Can you work these out from the model? Positions are in its coordinate system, mm. A direction names the side the tool comes from. Coordinates: 2 decimals unless noted, no trailing zeros. Order: outer loops, then holes, each group sorted by start corner. A loop starts at its lowest first (then second) coordinate and runs counter-clockwise, first axis right, second up. Notation, with made-up numbers: (24, 22) -> (52, 22) arc R9 cw to (52, 26) -> close; hole circle Ø3 at (-6, 85.5). An arc over 180 degrees is marked (long way). Answer as a JSON object with one key per item and string values. Group by question number.
(1) I need wall thicknesses on line 1 (X direction, y = 0.45, z = 34); line 2 (X direction, y = 1.6, z = -27); line 3 (Z direction, x = 20, y = 0.95). Which ranges of each line are inside material? Lowest first, please.
(2) I want a section at A-A, the plane z = -4. List the corners of the cut face in (x, y) for me.
(3) For pin 1 (0.8 mm diameter, centred on x = -1.5, y = 0.5, fed in from +Z); pin 2 (0.8 mm diameter, centred on x = 6, y = 2, fed in from -Z); pin 3 (0.8 mm diameter, centred on x = -21.5, z = 18, fed in from +Y), each with a flat end and sliding along its axis, tell me the tip position at first contact or that it passes through.
(4) I want a section at D-D, the plane x = -4.5. List the corners of the cut face in (y, z) for me.
(5) Which directions (+Z, -Z, +X, -X, +Y, -Y) give clear straight access to the entire face, cutting with the end or side of a thin tool? Please do faces 1 (the flat face through (-22, 1, -9)), 2 (the cylindrical face through (0.62, -1.4, -51.93)), 3 (the flat face through (24, 1, 0)).
(6) I want a section at B-B, the plane y = 0.8. List the corners of the cut face in (x, z) for me.
(7) I want a section at C-C, the plane z = -27.5. List the corners of the cut face in (x, y) for me.
(8) If we mould it in two halves opening along Z, with no side actions, what happens to faces 4 (the flat face through (22, 1, -11)), 5 (the flat face through (12, 1, -47)), 6 (the flat face through (-24, 1, -2))? For each: pulls with the +Z half, pulls with the -Z half, needs draft (parallel to the pull), parting line crosses it, or undercut.
from build123d import *

# Parameters (mm, degrees)
BOSS_EXTRUDE1_DEPTH = 2.5
SKETCH4_W           = 40
SKETCH4_H           = 1.5
BOSS_EXTRUDE3_DEPTH = 1.5
SKETCH6_R           = 2
BOSS_EXTRUDE4_DEPTH = 10


with BuildPart() as part:
    # Sketch2 → Boss-Extrude1 (new body)
    with BuildSketch(Plane(origin=(0, 0, 0), x_dir=(1, 0, 0), z_dir=(0, 1, 0))):
        Polygon((-22, -45), (-22, 45), (22, 45), (22, -45), (24, -45), (24, 47), (-24, 47), (-24, -45), align=None)
    extrude(amount=BOSS_EXTRUDE1_DEPTH)

    # Sketch4 → Boss-Extrude3 (add)
    with BuildSketch(Plane(origin=(-22, 0, 0), x_dir=(0, 0, -1), z_dir=(1, 0, 0))):
        Polygon((45, 1.75), (15, 1.75), (45, 2.5), align=None)
        with Locations((-25, 0.75)):
            Rectangle(SKETCH4_W, SKETCH4_H)
    boss_extrude3 = extrude(amount=BOSS_EXTRUDE3_DEPTH)

    # Mirror1: Boss-Extrude3 across plane
    add(boss_extrude3.mirror(Plane(origin=(0, 0, 0), x_dir=(0, 0, 1), z_dir=(1, 0, 0))))

    # Sketch6 → Boss-Extrude4 (add)
    with BuildSketch(Plane(origin=(0, 0, -47), x_dir=(-1, 0, 0), z_dir=(0, 0, -1))):
        with Locations(Location((0, 0.5, 0), (0, 0, 194.477512186))):
            Circle(SKETCH6_R)
    extrude(amount=BOSS_EXTRUDE4_DEPTH)


solid = part.part
Computed values:
{
 "1": {"line 1": "x = -24 to -20.5, 20.5 to 24", "line 2": "x = -24 to -22, 22 to 24", "line 3": "z = -47 to -45"},
 "2": {"outline": "(-24, 0) -> (-22, 0) -> (-22, 2.5) -> (-24, 2.5) -> close; (22, 0) -> (24, 0) -> (24, 2.5) -> (22, 2.5) -> close"},
 "3": {"pin 1": "stops at z = -45", "pin 2": "stops at z = -47", "pin 3": "stops at y = 1.5"},
 "4": {"outline": "(0, -47) -> (2.5, -47) -> (2.5, -45) -> (0, -45) -> close"},
 "5": {"face 1": "none", "face 2": "-Z", "face 3": "+Z, -Z, +X, +Y, -Y"},
 "6": {"outline": "(-24, -47) -> (-1.98, -47) -> (-1.98, -57) -> (1.98, -57) -> (1.98, -47) -> (24, -47) -> (24, 45) -> (20.5, 45) -> (20.5, 5) -> (22, 5) -> (22, -45) -> (-22, -45) -> (-22, 5) -> (-20.5, 5) -> (-20.5, 45) -> (-24, 45) -> close"},
 "7": {"outline": "(-24, 0) -> (-22, 0) -> (-22, 1.75) -> (-20.5, 1.75) -> (-20.5, 2.06) -> (-22, 2.06) -> (-22, 2.5) -> (-24, 2.5) -> close; (20.5, 1.75) -> (22, 1.75) -> (22, 0) -> (24, 0) -> (24, 2.5) -> (22, 2.5) -> (22, 2.06) -> (20.5, 2.06) -> close"},
 "8": {"face 4": "undercut", "face 5": "pulls with the -Z half", "face 6": "needs draft"}
}
